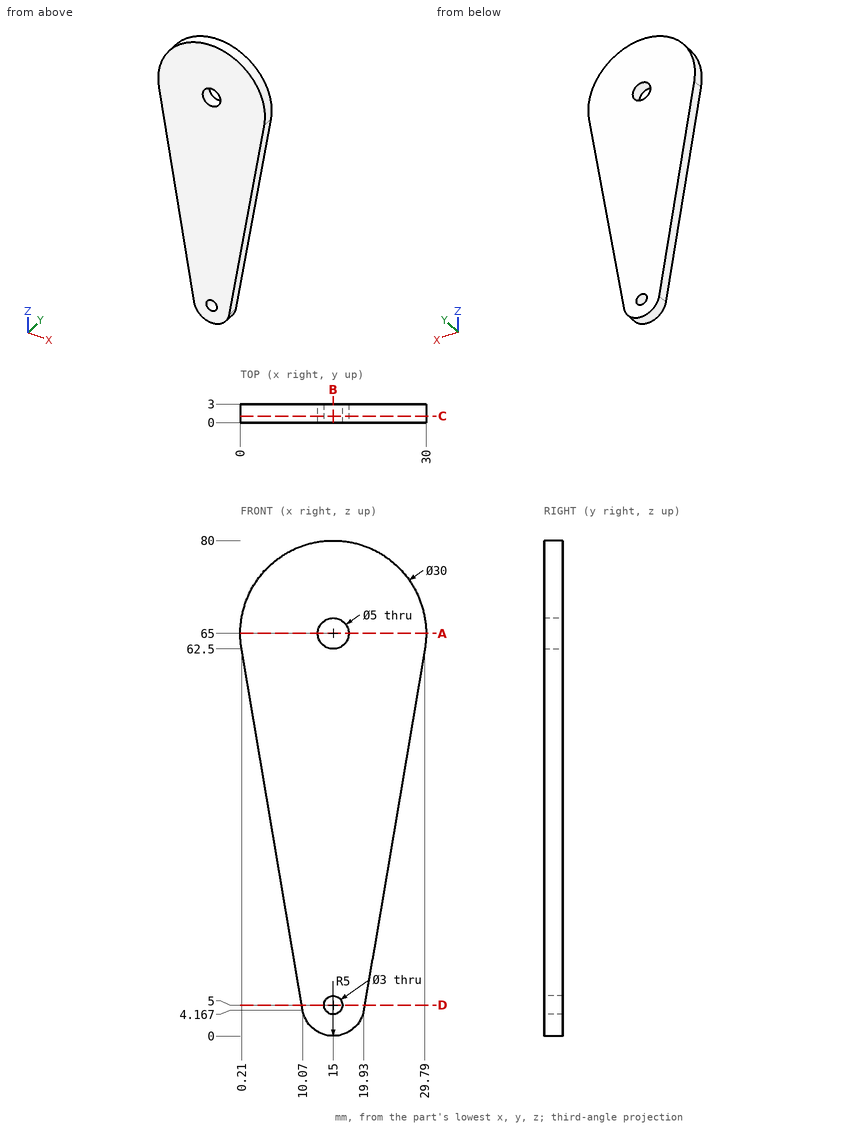
Source: three-view drawing plus pictorial views. Frame: mm from the lowest corner of the part. Give positions to 0.01 mm unless a question says otherwise; leave off trailing zeros. Write each loop counter-clockwise with the first axis right and the second up, starting at its lowest first coordinate (ties: lowest second). Pieces come first, ordered by that corner, then holes. Notation, with made-up numbers: (30.25, 78.5) -> (69.25, 78.5) arc R32 cw to (69.25, 108.5) -> close; hole circle Ø2 at (18.25, 72.5). An arc over 180 degrees is marked (long way). Write item = value, one per line.
Q1. Line query: line 1 (X direction, y = 1.25, z = 65); line 2 (Z direction, x = 16, y = 1.75) (1 decimal); line 3 (Z direction, x = 13, y = 0.6) (1 decimal). Output: solid intervals per line, ascending. Write a range as from..to.
Here are the results:
line_1 = 0..12.5, 17.5..30
line_2 = 0.1..3.9, 6.1..62.7, 67.3..80
line_3 = 0.4..63.5, 66.5..79.9
Q2. Cut plane B-B on x = 15. Return loops of the section in (y, z), then the cut area to 3 significant figures.
Here are the results:
outline = (0, 0) -> (3, 0) -> (3, 3.5) -> (0, 3.5) -> close; (0, 6.5) -> (3, 6.5) -> (3, 62.5) -> (0, 62.5) -> close; (0, 67.5) -> (3, 67.5) -> (3, 80) -> (0, 80) -> close
area = 216 mm²
Q3. Cut plane D-D on z = 5. Return loops of the section in (x, y).
Here are the results:
outline = (9.93, 0) -> (13.5, 0) -> (13.5, 3) -> (9.93, 3) -> close; (16.5, 0) -> (20.07, 0) -> (20.07, 3) -> (16.5, 3) -> close
Q4. First-contact query: pin 1 (1 mm diameter, centred on y = 1, z = 38.5, fed in from -X); pin 2 (1.5 mm diameter, centred on y = 2, z = 41, fed in from +X). Flat tips, straight axial feed; report the tip coordinate or a pass-through.
Here are the results:
pin_1 = 4.18
pin_2 = 26.28
Q5. Cut plane A-A on z = 65. Return loops of the section in (x, y), then the cut area to 3 significant figures.
Here are the results:
outline = (0, 0) -> (12.5, 0) -> (12.5, 3) -> (0, 3) -> close; (17.5, 0) -> (30, 0) -> (30, 3) -> (17.5, 3) -> close
area = 75.0 mm²
Q6. Cut plane C-C on y = 1.05. Return loops of the section in (x, z).
Here are the results:
outline = (0.21, 62.5) -> (10.07, 4.17) arc R5 ccw to (19.93, 4.17) -> (29.79, 62.5) arc R15 ccw (long way) to start; hole circle Ø5 at (15, 65); hole circle Ø3 at (15, 5)
